Work out the finished part from the listing and answer in its coordinate system (mm). Face numbers are marked on the shaded views. A direction names the side the tool comes from. Coordinates: 2 decimals unless noted, no trailing zeros. Write each loop counter-clockwise with the first axis right and the second up, starting at its lowest first coordinate (ties: lowest second). Pieces come first, ordered by that corner, then holes. Notation, with made-up numbers: (13, 71.25) - (65, 71.25) arc R25 cw to (65, 84.25) - close; hole circle Ø11 at (18, 72.5). An arc over 180 degrees is marked (long way). Use a Markdown table: item, result. Add a question column.
(1) The part is cut by section B-B, the plane z = 34.5. Give the vertices of the cut face in (x, y), then the cut area to 3 significant figures.
(2) Given pin 1 Ø1.5 at (x, z) = (-26, 39) entering from +Y; pin 2 Ø3 at (x, z) = (20.5, 73) entering from -Y; pin 3 Ø12 at (y, z) = (-25, 37) entering from +X; pin 4 Ø6 at (y, z) = (-25, 13.55) entering from -X, each flat-ended and moving along its own axis, determine where each tip first touches the part or whether it passes through.
(3) A tool of negligible diameter and unlimited length cuts with its end or side. For the marked faces 1 and 2, from which of +Z, -Z, +X, -X, +Y, -Y can it reach the whole face along a straight path? Write none if from no direction.
(4) Find the intervals of material crossed by line 1 (Z direction, x = -8, y = -25); line 2 (Z direction, x = -12.5, y = -21); line 3 (X direction, y = 29, z = 88), in increasing order. Write a range as from..to.
(5) The part is cut by section C-C, the plane x = -29.5. Give the vertices of the cut face in (y, z), then the cut area to 3 significant figures.
(6) The part is cut by section A-A, the plane y = -25. Give the vertices of the cut face in (x, z).
(7) The part is cut by section D-D, the plane x = -3. Give the vertices of the cut face in (y, z).
from build123d import *

# Parameters (mm, degrees)
F1_DEPTH = 93.548797
F3_D     = 10
F4_R     = 31
F5_SIZE  = 1
F6_R     = 5


with BuildPart() as f1:
    # F0 (on Top) → F1 (new body)
    with BuildSketch(Plane.XY):
        Polygon((50, -10), (-50, 50), (-50, -10), (0, -40), (0, -10), align=None)
    extrude(amount=F1_DEPTH)

    # F3 (through all)
    with Locations(Plane.YZ):
        with Locations((-25, 78.548797), (-25, 13.548797)):
            Hole(F3_D / 2)

    # F4
    f4_edges = [f1.edges().sort_by_distance(p)[0] for p in [
        (-50, -10, 46.774399),
    ]]
    fillet(f4_edges, radius=F4_R)

    # F5
    f5_edges = [f1.edges().sort_by_distance(p)[0] for p in [
        (0, -40, 46.774399),
    ]]
    chamfer(f5_edges, length=F5_SIZE)

    # F6
    f6_edges = [f1.edges().sort_by_distance(p)[0] for p in [
        (0, -10, 46.774399),
    ]]
    fillet(f6_edges, radius=F6_R)


solid = f1.part
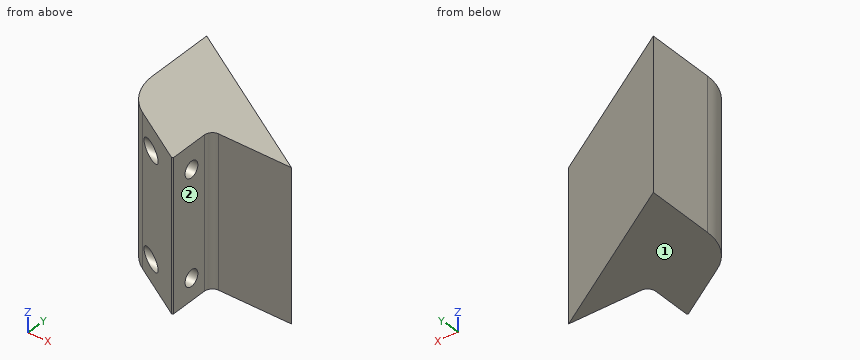
Model answer:
| question | item | result |
|---|---|---|
| 1 | outline | (-50, 7.55) arc R31 ccw to (-34.95, -19.03) - (-0.86, -39.49) - (0, -39) - (0, -15) arc R5 cw to (5, -10) - (50, -10) - (-50, 50) - close |
| 1 | area | 3,710 mm^2 |
| 2 | pin 1 | y = 36.05 |
| 2 | pin 2 | y = -10 |
| 2 | pin 3 | x = 0 |
| 2 | pin 4 | through |
| 3 | face 1 | -Z, +X, -X, +Y, -Y |
| 3 | face 2 | +Z, -Z, +X, -Y |
| 4 | line 1 | 0..8.55, 18.55..73.55, 83.55..93.55 |
| 4 | line 2 | 0..10.55, 16.55..75.55, 81.55..93.55 |
| 4 | line 3 | -50..-15 |
| 5 | outline | (-22.3, 0) - (37.7, 0) - (37.7, 93.55) - (-22.3, 93.55) - (-22.3, 82.76) arc R5 cw to (-22.3, 74.34) - (-22.3, 17.76) arc R5 cw to (-22.3, 9.34) - close |
| 5 | area | 5,590 mm^2 |
| 6 | outline | (-25, 0) - (0, 0) - (0, 8.55) - (-25, 8.55) - close; (-25, 18.55) - (0, 18.55) - (0, 73.55) - (-25, 73.55) - close; (-25, 83.55) - (0, 83.55) - (0, 93.55) - (-25, 93.55) - close |
| 7 | outline | (-38.2, 0) - (21.8, 0) - (21.8, 93.55) - (-38.2, 93.55) - close; hole circle Ø10 at (-25, 13.55); hole circle Ø10 at (-25, 78.55) |
